Verification items for the finished model (mm, model axes). A direction names the side the tool comes from. Round coordinates to 2 decimals unless told otherwise and drop trailing zeros. Return JSON: item names as keys, results as strings. Group by question number.
1) Draft check along X on faces 1 (the flat face through (35, 51, 70)), 2 (the flat face through (40, 10, 20)), 3 (the flat face through (0, 49, 35)), 4 (the cylindrical face through (40, 5, 22)). Enter one of: pulls with the +X half, pulls with the -X half, needs draft (parallel to the pull), parting line crosses it, or undercut.
2) Tool access check on faces 5 (the flat face through (35, 0, 35)), 6 (the flat face through (40, 10, 50)). Record the directions out of +Z, -Z, +X, -X, +Y, -Y that give a thin tool (end or side, any length) a straight path to the whole face; none if there is none.
3) Depth check by flat-ended pin: pin 1 (1.2 mm diameter, centred on x = 40.5, z = 49.5, fed in from -Y). Enter the tip coordinate at first touch or a pass-through.
4) Scan line: L1, parallel to Z at x = 40, y = 3.5. Record every from-to range of solid material in increasing order.
```python
from build123d import *

# Parameters (mm, degrees)
SKETCH_1_W          = 72
SKETCH_1_H          = 100
EXTRUDE_1_DEPTH     = 70
SKETCH_2_R          = 2
CUT_EXTRUDE_1_DEPTH = 10


with BuildPart() as part:
    # Эскиз1 → Бобышка-Вытянуть1 (new body)
    with BuildSketch(Plane.XY):
        with Locations((36, 50)):
            Rectangle(SKETCH_1_W, SKETCH_1_H)
    extrude(amount=EXTRUDE_1_DEPTH)

    # Эскиз2 → Вырез-Вытянуть1 (cut)
    with BuildSketch(Plane.XZ):
        with Locations((40, 50)):
            Circle(SKETCH_2_R)
        with Locations((40, 20)):
            Circle(SKETCH_2_R)
    extrude(amount=-CUT_EXTRUDE_1_DEPTH, mode=Mode.SUBTRACT)


solid = part.part
```
Check result:
{
 "1": {"face 1": "needs draft", "face 2": "undercut", "face 3": "pulls with the -X half", "face 4": "undercut"},
 "2": {"face 5": "+Z, -Z, +X, -X, -Y", "face 6": "-Y"},
 "3": {"pin 1": "y = 10"},
 "4": {"L1": "0 to 18, 22 to 48, 52 to 70"}
}
